Verification items for the finished model (mm, model axes). A direction names the side the tool comes from. Round coordinates to 2 decimals unless told otherwise and drop trailing zeros. Write each loop counter-clockwise with the first axis right and the second up, starting at its lowest first coordinate (ties: lowest second). Pieces come first, ordered by that corner, then holes. Notation, with made-up numbers: M 75,69.25 L 103,69.25 A4 cw 103,76.25 Z; hole C -6,23.5 d1. An arc over 180 degrees is marked long. One line per item, written item: value. Start each with the question number.
Item 1: Thickness scan on probe 1 along Z at (x, y) = (0, 3.2); probe 2 along X at (y, z) = (1.45, 0); probe 3 along Z at (x, y) = (0, 1.15). Record the ranges inside material, lowest first. Write a range as from..to.
Item 2: Section check D-D, the plane y = 1.25. Record the cut outline in (x, z).
Item 3: Tool access check on faces 4 (the face through (-10.864, 2.071, 3.154)), 5 (the face through (-2, 2.9, -7)), 6 (the face through (8.16, 2.07, 7.83)), 7 (the face through (-8.21, 2.07, 7.86)). Record the directions out of +Z, -Z, +X, -X, +Y, -Y that give a thin tool (end or side, any length) a straight path to the whole face; none if there is none.
Item 4: Draft check along X on faces 1 (the face through (-9, 4.2, -5)), 2 (the face through (-11.6, 2.07, -6.51)), 3 (the face through (2.7, 2, -11)). Enter one of: +X half, -X half, draft (parallel to the pull), parting line (faces both ways), or undercut.
Item 5: Gauge pin test, flat ends, axial feed: pin 1 (2 mm diameter, centred on y = 2.5, z = -11.5, fed in from +X); pin 2 (1.2 mm diameter, centred on y = 2.5, z = -11, fed in from -X); pin 3 (1.5 mm diameter, centred on x = -6, y = 0.5, fed in from -Z). Record the tip position at first contact, or that the pin passes through.
Item 6: Section check C-C, the plane y = 3.5. Record the cut outline in (x, z), then the cut area to 3 significant figures.
Item 7: Section check B-B, the plane z = -1.75. Record the cut outline in (x, y), then the cut area to 3 significant figures.
Item 8: Section check A-A, the plane x = 0. Record the cut outline in (y, z), then the cut area to 3 significant figures.
Autodesk Fusion 360 part; units mm, degrees
sketch "Esboço1" plane through (0, 0, 0) normal (0, 1, 0) x (1, 0, 0)
  circle A0 centre (0, 0) radius 13.3
  circle A1 centre (0, 0) radius 9.4
  circle A2 centre (0, 0) radius 7.1
  circle A3 centre (0, 0) radius 5.75
  line L0 (-2.7, 13.0231) -> (-2.7, 9.0039)
  line L1 (2.7, 9.0039) -> (2.7, 13.0231)
  line L2 (0, 0) -> (0, 16.7513) construction
  line L3 (-9.9283, -8.8498) -> (-6.4476, -6.8402)
  line L4 (-9.1476, -2.1637) -> (-12.6283, -4.1733)
  line L5 (12.6283, -4.1733) -> (9.1476, -2.1637)
  line L6 (6.4476, -6.8402) -> (9.9283, -8.8498)
  dimension "d1" = 11.5
  dimension "d2" = 14.2
  dimension "d3" = 18.8
  dimension "d4" = 26.6
  dimension "d5" = 5.4
  dimension "d6" = 2.7
  dimension "d8" = 360
extrude "Extrusão1" add sketch "Esboço1" along normal blind 4.2 contours A0 A1 L1 L5 | A0 A1 L0 L4 | A0 A1 L3 L6 | A2 makes body 1 at (12.9632, 2.8, 2.9742) makes body 2 at (7.0647, 1.4, 0.7069) makes body 3 at (6.551, 2.8, 11.5747) makes body 4 at (-12.8098, 2.8, 3.5776)
extrude "Extrusão2" add sketch "Esboço1" along normal blind 2.9 contours A1 bodies 1 2 3 4
Response values:
1. probe 1: z = -7.1..-5.75, 5.75..7.1, 9.4..13.3
1. probe 2: x = -13.3..-5.75, 5.75..13.3
1. probe 3: z = -9.4..-5.75, 5.75..13.3
2. outline: M -12.63,4.17 A13.3 ccw -2.7,-13.02 L -2.7,-9 A9.4 ccw 2.7,-9 L 2.7,-13.02 A13.3 ccw 12.63,4.17 L 9.15,2.16 A9.4 ccw 6.45,6.84 L 9.93,8.85 A13.3 ccw -9.93,8.85 L -6.45,6.84 A9.4 ccw -9.15,2.16 Z; hole C 0,0 d11.5
3. face 4: +Y, -Y
3. face 5: +Y
3. face 6: +X, +Y, -Y
3. face 7: -X, +Y, -Y
4. face 1: draft
4. face 2: -X half
4. face 3: undercut
5. pin 1: stops at x = 8.16
5. pin 2: stops at x = -8.29
5. pin 3: stops at z = -12.22
6. outline: M -12.63,4.17 A13.3 ccw -2.7,-13.02 L -2.7,-9 A9.4 cw -9.15,2.16 Z; M -9.93,8.85 L -6.45,6.84 A9.4 cw 6.45,6.84 L 9.93,8.85 A13.3 ccw Z; C 0,0 d14.2; M 2.7,-13.02 A13.3 ccw 12.63,4.17 L 9.15,2.16 A9.4 cw 2.7,-9 Z; hole C 0,0 d11.5
6. area: 269 mm2
7. outline: M -13.18,0 L -5.48,0 L -5.48,4.2 L -6.88,4.2 L -6.88,2.9 L -9.24,2.9 L -9.24,4.2 L -13.18,4.2 Z; M 5.48,0 L 13.18,0 L 13.18,4.2 L 9.24,4.2 L 9.24,2.9 L 6.88,2.9 L 6.88,4.2 L 5.48,4.2 Z
7. area: 58.6 mm2
8. outline: M 0,-9.4 L 2.9,-9.4 L 2.9,-7.1 L 4.2,-7.1 L 4.2,-5.75 L 0,-5.75 Z; M 0,5.75 L 4.2,5.75 L 4.2,7.1 L 2.9,7.1 L 2.9,9.4 L 4.2,9.4 L 4.2,13.3 L 0,13.3 Z
8. area: 41.1 mm2
